from build123d import *

# Parameters (mm, degrees)
F1_DEPTH = 76.2
F2_W     = 25.4
F2_H     = 63.5
F3_DEPTH = 114.3
F5_DEPTH = 25.4


with BuildPart() as f1:
    # F0 (on Front) → F1 (new body)
    with BuildSketch(Plane.XZ):
        Polygon((-23.121473, 14.273803), (-23.121473, -49.226197), (40.378527, -49.226197), (14.978527, 14.273803), align=None)
    extrude(amount=F1_DEPTH)

    # F2 (on face) → F3 (join)
    with BuildSketch(Plane(origin=(-23.121473, 0, 0), x_dir=(0, -1, 0), z_dir=(-1, 0, 0))):
        with Locations((38.1, -17.476197)):
            Rectangle(F2_W, F2_H)
    extrude(amount=-F3_DEPTH)

    # F4 (on face) → F5 (cut)
    with BuildSketch(Plane(origin=(0, -25.4, 0), x_dir=(-1, 0, 0), z_dir=(0, 1, 0))):
        Polygon((-91.178527, -49.226197), (-65.778527, 14.273803), (-91.178527, 14.273803), align=None)
    extrude(amount=-F5_DEPTH, mode=Mode.SUBTRACT)


solid = f1.part
Here's how the part is built. I have some questions about the finished solid (model axes, mm). A direction names the side the tool comes from. Give positions to 0.01 mm unless a question says otherwise; leave off trailing zeros. Loops run counter-clockwise (first coordinate to the right, second up) from the corner with the lowest first, then second, coordinate; pieces in that order, holes last. Notation, with made-up numbers: (48.25, -19.75) -> (97.25, -19.75) arc R22 cw to (97.25, -7.75) -> close; hole circle Ø10 at (61.25, 63.5). An arc over 180 degrees is marked (long way). Answer as a JSON object with one key per item and string values. Group by question number.
Item 1: I need wall thicknesses on L1, parallel to Y at x = 87, z = -41.5; L2, parallel to X at y = -54.5, z = -20.5; L3, parallel to X at y = -28, z = -16. Which ranges of each line are inside material? Lowest first, please.
Item 2: Imagine slicing it at C-C on y = -27. Write out the boundary of the cut face in (x, z), then the cut area to 3 significant figures.
Item 3: Will these pins go through, and if not, where does the flat tip stop? pin 1 (4 mm diameter, centred on x = 1, z = -20, fed in from +Y); pin 2 (1 mm diameter, centred on y = -10, z = -19, fed in from +X); pin 3 (19 mm diameter, centred on x = 71, z = -9, fed in from +Y); pin 4 (1 mm diameter, centred on y = -26, z = -5.5, fed in from +X).
Item 4: On a 3-axis mill with a long thin cutter (end or side, diameter ignored), from which of +Z, -Z, +X, -X, +Y, -Y can I reach the whole of each face in a straight line? I mean faces 1 (the flat face through (53, -50.8, -18)), 2 (the flat face through (53, -25.4, -18)), 3 (the flat face through (1, -76.2, -17)). Say none if no direction works.
Item 5: Imagine slicing it at B-B on x = 59. Write out the boundary of the cut face in (y, z), then the cut area to 3 significant figures.
Item 6: Imagine slicing it at A-A on z = 10.5. Write out the boundary of the cut face in (x, y).
Item 7: Imagine slicing it at D-D on z = -15.5. Write out the boundary of the cut face in (x, y).
Answer list:
{
 "1": {"L1": "y = -50.8 to -25.4", "L2": "x = -23.12 to 28.89", "L3": "x = -23.12 to 77.89"},
 "2": {"outline": "(-23.12, -49.23) -> (91.18, -49.23) -> (65.78, 14.27) -> (-23.12, 14.27) -> close", "area": "6,450 mm2"},
 "3": {"pin 1": "stops at y = 0", "pin 2": "stops at x = 28.49", "pin 3": "stops at y = -25.4", "pin 4": "stops at x = 73.89"},
 "4": {"face 1": "+Z, +X, -Y", "face 2": "+Z, +X, +Y", "face 3": "+Z, -Z, +X, -X, -Y"},
 "5": {"outline": "(-50.8, -49.23) -> (-25.4, -49.23) -> (-25.4, 14.27) -> (-50.8, 14.27) -> close", "area": "1,610 mm2"},
 "6": {"outline": "(-23.12, -76.2) -> (16.49, -76.2) -> (16.49, -50.8) -> (67.29, -50.8) -> (67.29, -25.4) -> (16.49, -25.4) -> (16.49, 0) -> (-23.12, 0) -> close"},
 "7": {"outline": "(-23.12, -76.2) -> (26.89, -76.2) -> (26.89, -50.8) -> (77.69, -50.8) -> (77.69, -25.4) -> (26.89, -25.4) -> (26.89, 0) -> (-23.12, 0) -> close"}
}
